```python
from build123d import *

# Parameters (mm, degrees)
SKETCH_1_W             = 350
SKETCH_1_H             = 300
EXTRUDE_1_DEPTH        = 20
FILLET_1_R             = 9
CUT_EXTRUDE_1_DEPTH    = 1
HOLE_WIZARD_M6_1_D     = 5
HOLE_WIZARD_M6_1_DEPTH = 14
HOLE_WIZARD_M6_1_TIP   = 1.502151548
HOLE_WIZARD_M6_2_D     = 5
HOLE_WIZARD_M6_2_DEPTH = 12
HOLE_WIZARD_M6_2_TIP   = 1.502151548


with BuildPart() as part:
    # 스케치1 → 보스-돌출1 (new body)
    with BuildSketch(Plane(origin=(0, 0, 0), x_dir=(1, 0, 0), z_dir=(0, 1, 0))):
        Rectangle(SKETCH_1_W, SKETCH_1_H)
    extrude(amount=EXTRUDE_1_DEPTH)

    # 필렛1
    fillet_1_edges = [part.edges().sort_by_distance(p)[0] for p in [
        (175, 10, 150),
        (-175, 10, 150),
        (-175, 10, -150),
        (175, 10, -150),
    ]]
    fillet(fillet_1_edges, radius=FILLET_1_R)

    # 스케치2 → 컷-돌출1 (cut)
    with BuildSketch(Plane(origin=(0, 20, 0), x_dir=(1, 0, 0), z_dir=(0, 1, 0))):
        with BuildLine():
            Line((-131, -150), (-50, -150))
            Line((-50, -150), (-50, -122))
            ThreePointArc((-50, -122), (-51.464466094, -118.464466094), (-55, -117))
            Line((-55, -117), (-126, -117))
            ThreePointArc((-126, -117), (-129.535533906, -118.464466094), (-131, -122))
            Line((-131, -122), (-131, -150))
        make_face()
        with BuildLine():
            Line((50, -150), (131, -150))
            Line((131, -150), (131, -122))
            ThreePointArc((131, -122), (129.535533906, -118.464466094), (126, -117))
            Line((126, -117), (55, -117))
            ThreePointArc((55, -117), (51.464466094, -118.464466094), (50, -122))
            Line((50, -122), (50, -150))
        make_face()
    extrude(amount=-CUT_EXTRUDE_1_DEPTH, mode=Mode.SUBTRACT)

    # M6 나사 구멍1
    with Locations(Plane(origin=(0, 19, 0), x_dir=(1, 0, 0), z_dir=(0, 1, 0))):
        with Locations((-110.5, -132.5), (-70.5, -132.5), (70.5, -132.5), (110.5, -132.5)):
            Hole(HOLE_WIZARD_M6_1_D / 2, depth=HOLE_WIZARD_M6_1_DEPTH)
            with Locations((0, 0, -(HOLE_WIZARD_M6_1_DEPTH + HOLE_WIZARD_M6_1_TIP / 2))):  # 118° drill point
                Cone(0, HOLE_WIZARD_M6_1_D / 2, HOLE_WIZARD_M6_1_TIP, mode=Mode.SUBTRACT)

    # M6 나사 구멍2
    with Locations(Plane(origin=(0, 20, 0), x_dir=(1, 0, 0), z_dir=(0, 1, 0))):
        with Locations((-62.5, 120), (62.5, 120)):
            Hole(HOLE_WIZARD_M6_2_D / 2, depth=HOLE_WIZARD_M6_2_DEPTH)
            with Locations((0, 0, -(HOLE_WIZARD_M6_2_DEPTH + HOLE_WIZARD_M6_2_TIP / 2))):  # 118° drill point
                Cone(0, HOLE_WIZARD_M6_2_D / 2, HOLE_WIZARD_M6_2_TIP, mode=Mode.SUBTRACT)


solid = part.part
```
The listing builds one solid part. Answer for the finished solid, in the listing's coordinates (mm). A direction names the side the tool comes from. Round coordinates to 2 decimals unless told otherwise and drop trailing zeros.
Q1. Which of the six approach directions +Z, -Z, +X, -X, +Y, -Y give full straight-line access (tool end or side, diameter ignored) to faces 1 (the face through (-91, 19, 133)), 2 (the face through (-172.434, 10.14, -147.294))?
Q2. Find the intervals of material crossed by line 1 (X direction, y = 9, z = 132.5); line 2 (Z direction, x = 110.5, y = 8.25); line 3 (Z direction, x = -62.5, y = 15.25), in increasing order.
Q3. Given pin 1 Ø3 at (x, z) = (70.5, 132.5) entering from +Y; pin 2 Ø4 at (x, z) = (-110.5, 132.5) entering from +Y; pin 3 Ø3 at (x, z) = (-62.5, -120) entering from +Y, each flat-ended and moving along its own axis, determine where each tip first touches the part or whether it passes through.
Completed:
1. face 1: +Z, +Y
1. face 2: -Z, -X, +Y, -Y
2. line 1: x = -175 to -113, -108 to -73, -68 to 68, 73 to 108, 113 to 175
2. line 2: z = -150 to 130, 135 to 150
2. line 3: z = -150 to -122.5, -117.5 to 150
3. pin 1: stops at y = 4.4
3. pin 2: stops at y = 4.7
3. pin 3: stops at y = 7.4
